Could you check a few things on this model? Use its own coordinates, in mm. A direction names the side the tool comes from. Round coordinates to 2 decimals unless told otherwise and drop trailing zeros. Loops run counter-clockwise (first coordinate to the right, second up) from the corner with the lowest first, then second, coordinate; pieces in that order, holes last. Notation, with made-up numbers: (35, 34.25) - (51, 34.25) arc R35 ccw to (51, 69.25) - close; hole circle Ø11 at (6.5, 54.5). An arc over 180 degrees is marked (long way). Answer as CSV lines item,"result". Start each with the question number.
1) We'd pull the mould along Z, two halves only. Please class faces 3 (the face through (5.062, 7.395, 0.665)), 4 (the face through (8.47, 0.99, 9.83)), 5 (the face through (-14.871, 0.987, -7.796)): pulls with the +Z half, pulls with the -Z half, needs draft (parallel to the pull), parting line crosses it, or undercut.
2) I'm going to push flat-ended pins straight in: pin 1 Ø6 at (y, z) = (14, -7) entering from -X; pin 2 Ø1 at (x, z) = (9.5, 0.5) entering from +Y; pin 3 Ø6 at (x, y) = (0.5, 11.5) entering from -Z. Where does each tip first touch, or does it pass through?
3) Suppose I cut it at C-C, the plane y = 5.25. Write out the boundary of the cut face in (x, z) (3 decimals), then the cut area to 3 significant figures.
4) Suppose I cut it at B-B, the plane z = 0. Write out the boundary of the cut face in (x, y) (3 decimals), then the cut area to 3 significant figures.
5) Which directions (+Z, -Z, +X, -X, +Y, -Y) give clear straight access to the entire face, cutting with the end or side of a thin tool? Please do faces 1 (the face through (-2.824, 9.409, -8.966)), 2 (the face through (-0.04, 0.99, 11.75)).
6) Please list where these lines run through material, in increasing order: line 1 along X through (y, z) = (7.5, 0) (3 decimals); line 2 along X through (y, z) = (16.05, 0); line 3 along Y through (x, z) = (-14, -1).
7) Suppose I cut it at A-A, the plane x = 0. Write out the boundary of the cut face in (y, z) (3 decimals), then the cut area to 3 significant figures.
```python
from build123d import *

# Parameters (mm, degrees)
BOSS_EXTRUDE3_DEPTH = 2
SKETCH2_R           = 9.4
BOSS_EXTRUDE2_DEPTH = 15
SKETCH3_R           = 5.105
CUT_EXTRUDE1_DEPTH  = 15
SKETCH4_R           = 3.75
CUT_EXTRUDE2_DEPTH  = 26.535514485
FILLET2_R           = 1
FILLET4_R           = 0.1


with BuildPart() as part:
    # Sketch6 → Boss-Extrude3 (new body)
    with BuildSketch(Plane(origin=(0, 0, 0), x_dir=(1, 0, 0), z_dir=(0, 1, 0))):
        with BuildLine():
            Line((-3.16984511, 11.314352919), (-13.922193144, 8.301959893))
            ThreePointArc((-13.922193144, 8.301959893), (-14.882365074, 7.78622676), (-15.531854224, 6.910969857))
            ThreePointArc((-15.531854224, 6.910969857), (-17, 0), (-15.531854224, -6.910969857))
            ThreePointArc((-15.531854224, -6.910969857), (-14.882365074, -7.78622676), (-13.922193144, -8.301959893))
            Line((-13.922193144, -8.301959893), (-3.16984511, -11.314352919))
            ThreePointArc((-3.16984511, -11.314352919), (0, -11.75), (3.16984511, -11.314352919))
            Line((3.16984511, -11.314352919), (13.922193144, -8.301959893))
            ThreePointArc((13.922193144, -8.301959893), (14.882365074, -7.78622676), (15.531854224, -6.910969857))
            ThreePointArc((15.531854224, -6.910969857), (17, 0), (15.531854224, 6.910969857))
            ThreePointArc((15.531854224, 6.910969857), (14.882365074, 7.78622676), (13.922193144, 8.301959893))
            Line((13.922193144, 8.301959893), (3.16984511, 11.314352919))
            ThreePointArc((3.16984511, 11.314352919), (0, 11.75), (-3.16984511, 11.314352919))
        make_face()
    extrude(amount=BOSS_EXTRUDE3_DEPTH)

    # Sketch2 → Boss-Extrude2 (add)
    with BuildSketch(Plane(origin=(0, 2, 0), x_dir=(1, 0, 0), z_dir=(0, 1, 0))):
        with Locations(Location((0, 0, 0), (0, 0, 90))):
            Circle(SKETCH2_R)
    extrude(amount=BOSS_EXTRUDE2_DEPTH)

    # Sketch3 → Cut-Extrude1 (cut)
    with BuildSketch(Plane.XZ):
        with Locations(Location((0, 0, 0), (0, 0, 270))):
            Circle(SKETCH3_R)
    extrude(amount=-CUT_EXTRUDE1_DEPTH, mode=Mode.SUBTRACT)

    # Sketch4 → Cut-Extrude2 (cut, through all)
    with BuildSketch(Plane.XZ.offset(-15)):
        with Locations(Location((0, 0, 0), (0, 0, 270))):
            Circle(SKETCH4_R)
    extrude(amount=-CUT_EXTRUDE2_DEPTH, mode=Mode.SUBTRACT)

    # Fillet2
    fillet2_edges = [part.edges().sort_by_distance(p)[0] for p in [
        (0, 2, 9.4),
        (0, 17, 9.4),
    ]]
    fillet(fillet2_edges, radius=FILLET2_R)

    # Fillet4
    fillet4_edges = [part.edges().sort_by_distance(p)[0] for p in [
        (0, 2, -11.75),
        (17, 0, 0),
        (14.882365074, 0, 7.78622676),
        (8.546019127, 0, 9.808156406),
        (0, 0, 11.75),
        (-8.546019127, 0, 9.808156406),
        (-14.882365074, 0, 7.78622676),
        (-8.546019127, 2, -9.808156406),
        (-17, 0, 0),
        (-14.882365074, 0, -7.78622676),
        (-8.546019127, 0, -9.808156406),
        (0, 0, -11.75),
        (8.546019127, 0, -9.808156406),
        (14.882365074, 0, -7.78622676),
        (-14.882365074, 2, -7.78622676),
        (-17, 2, 0),
        (-14.882365074, 2, 7.78622676),
        (-8.546019127, 2, 9.808156406),
        (0, 2, 11.75),
        (8.546019127, 2, 9.808156406),
        (14.882365074, 2, 7.78622676),
        (17, 2, 0),
        (14.882365074, 2, -7.78622676),
        (8.546019127, 2, -9.808156406),
    ]]
    fillet(fillet4_edges, radius=FILLET4_R)


solid = part.part
```
Filled sheet:
1,face 3,"undercut"
1,face 4,"pulls with the +Z half"
1,face 5,"pulls with the -Z half"
2,pin 1,"x = -8.51"
2,pin 2,"y = 16.79"
2,pin 3,"z = -9.4"
3,outline,"circle Ø18.8 at (0, 0); hole circle Ø10.21 at (0, 0)"
3,area,"196 mm²"
4,outline,"(-17, 0.1) arc R0.1 ccw to (-16.9, 0) - (-5.105, 0) - (-5.105, 15) - (-3.75, 15) - (-3.75, 17) - (-8.4, 17) arc R1 ccw to (-9.4, 16) - (-9.4, 3) arc R1 cw to (-10.4, 2) - (-16.9, 2) arc R0.1 ccw to (-17, 1.9) - close; (3.75, 15) - (5.105, 15) - (5.105, 0) - (16.9, 0) arc R0.1 ccw to (17, 0.1) - (17, 1.9) arc R0.1 ccw to (16.9, 2) - (10.4, 2) arc R1 cw to (9.4, 3) - (9.4, 16) arc R1 ccw to (8.4, 17) - (3.75, 17) - close"
4,area,"182 mm²"
5,face 1,"+Y"
5,face 2,"+Z, +Y, -Y"
6,line 1,"-9.4 to -5.105, 5.105 to 9.4"
6,line 2,"-9.4 to -3.75, 3.75 to 9.4"
6,line 3,"0 to 2"
7,outline,"(0, -11.65) arc R0.1 ccw to (0.1, -11.75) - (1.9, -11.75) arc R0.1 ccw to (2, -11.65) - (2, -10.4) arc R1 cw to (3, -9.4) - (16, -9.4) arc R1 ccw to (17, -8.4) - (17, -3.75) - (15, -3.75) - (15, -5.105) - (0, -5.105) - close; (0, 5.105) - (15, 5.105) - (15, 3.75) - (17, 3.75) - (17, 8.4) arc R1 ccw to (16, 9.4) - (3, 9.4) arc R1 cw to (2, 10.4) - (2, 11.65) arc R0.1 ccw to (1.9, 11.75) - (0.1, 11.75) arc R0.1 ccw to (0, 11.65) - close"
7,area,"161 mm²"
